Design review of the part built by this model. Coordinates are the model's own, in mm. Round coordinates to 2 decimals unless told otherwise and drop trailing zeros. Write each loop counter-clockwise with the first axis right and the second up, starting at its lowest first coordinate (ties: lowest second). Pieces come first, ordered by that corner, then holes. Notation, with made-up numbers: (8.25, 13) -> (66.25, 13) arc R17 ccw to (66.25, 26) -> close; hole circle Ø10 at (61.25, 53). An arc over 180 degrees is marked (long way). Write item = value, one per line. Start each with the question number.
Item 1: Add section A-A, the plane y = 27.75. State the section outline as (x, z) points.
Item 2: To check wall thickness, follow L1, parallel to Y at x = 9.44, z = 7.5. State the ranges of the line that lie inside material, in increasing order.
Item 3: Add section B-B, the plane x = -9.44. State the section outline as (y, z) points.
Item 4: Mouldability with a two-part tool opening along Y and no side actions: class faces 1 (the flat face through (0, 0, 0)), 2 (the cylindrical face through (8.25, -28.13, 7.1)), 3 (the flat face through (0, 31.05, 7)) as released by +Y, released by -Y, zero draft, split by the parting line, or undercut.
from build123d import *

# Parameters (mm, degrees)
SKETCH_1_W      = 25.48
SKETCH_1_H      = 62.1
SKETCH_1_R      = 1.25
EXTRUDE_1_DEPTH = 14.41


with BuildPart() as part:
    # 草圖1 → 填料-伸長1 (new body)
    with BuildSketch(Plane.XY):
        Rectangle(SKETCH_1_W, SKETCH_1_H)
        with Locations((9.44, 27.75)):
            Circle(SKETCH_1_R, mode=Mode.SUBTRACT)
        with Locations(Location((-9.44, 27.75, 0), (0, 0, 180))):
            Circle(SKETCH_1_R, mode=Mode.SUBTRACT)
        with Locations(Location((9.44, -27.75, 0), (0, 0, 180))):
            Circle(SKETCH_1_R, mode=Mode.SUBTRACT)
        with Locations((-9.44, -27.75)):
            Circle(SKETCH_1_R, mode=Mode.SUBTRACT)
    extrude(amount=EXTRUDE_1_DEPTH)


solid = part.part
Result set:
q1.outline = (-12.74, 0) -> (-10.69, 0) -> (-10.69, 14.41) -> (-12.74, 14.41) -> close; (-8.19, 0) -> (8.19, 0) -> (8.19, 14.41) -> (-8.19, 14.41) -> close; (10.69, 0) -> (12.74, 0) -> (12.74, 14.41) -> (10.69, 14.41) -> close
q2.L1 = -31.05 to -29, -26.5 to 26.5, 29 to 31.05
q3.outline = (-31.05, 0) -> (-29, 0) -> (-29, 14.41) -> (-31.05, 14.41) -> close; (-26.5, 0) -> (26.5, 0) -> (26.5, 14.41) -> (-26.5, 14.41) -> close; (29, 0) -> (31.05, 0) -> (31.05, 14.41) -> (29, 14.41) -> close
q4.face_1 = zero draft
q4.face_2 = undercut
q4.face_3 = released by +Y
